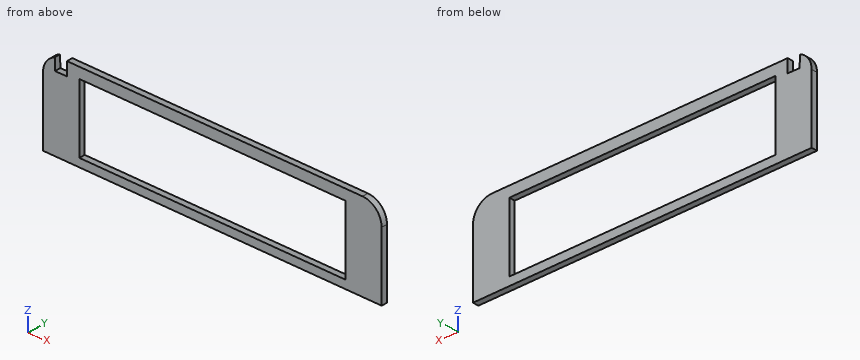
```python
from build123d import *

# Parameters (mm, degrees)
F0_W     = 70.612
F0_H     = 18.034
F1_DEPTH = 1.5748


with BuildPart() as f1:
    # F0 (on Front) → F1 (new body)
    with BuildSketch(Plane.XZ):
        with BuildLine():
            Line((43.006146, 12.59901), (-35.475917, 12.59901))
            Line((-35.475917, 12.59901), (-35.423273, 9.108076))
            Line((-35.423273, 9.108076), (-38.651996, 9.059386))
            Line((-38.651996, 9.059386), (-38.69928, 12.194926))
            ThreePointArc((-38.69928, 12.194926), (-40.974954, 10.332579), (-41.829854, 7.51901))
            Line((-41.829854, 7.51901), (-41.829854, -10.40099))
            Line((-41.829854, -10.40099), (48.086146, -10.40099))
            Line((48.086146, -10.40099), (48.086146, 7.51901))
            ThreePointArc((48.086146, 7.51901), (46.598248, 11.111112), (43.006146, 12.59901))
        make_face()
        with Locations((3.128146, 0.78801)):
            Rectangle(F0_W, F0_H, mode=Mode.SUBTRACT)
    extrude(amount=F1_DEPTH)


solid = f1.part
```
The model under review builds one solid part; all positions refer to its coordinate system, in mm. Round coordinates to 2 decimals unless told otherwise and drop trailing zeros. Loops run counter-clockwise (first coordinate to the right, second up) from the corner with the lowest first, then second, coordinate; pieces in that order, holes last. Notation, with made-up numbers: M 21,1 L 65,1 A36 ccw 65,37 Z; hole C 6,7 d4. An arc over 180 degrees is marked long. Put each result on its own line as item: value.
Q1. Consider section C-C, the plane y = -1.1. Give the boundary of the cut face in (x, z) (3 decimals), then the cut area to 3 significant figures.
Result set:
outline: M -41.83,-10.401 L 48.086,-10.401 L 48.086,7.519 A5.08 ccw 43.006,12.599 L -35.476,12.599 L -35.423,9.108 L -38.652,9.059 L -38.699,12.195 A5.057 ccw -41.83,7.519 Z; hole M -32.178,-8.229 L 38.434,-8.229 L 38.434,9.805 L -32.178,9.805 Z
area: 772 mm²
Q2. To check wall thickness, follow L1, parallel to X at y = -0.05, z = -7.5; L2, parallel to Z at x = -21, y = -1.05; L3, parallel to X at y = -0.25, z = 11.75. State the ranges of each line that lie inside material, in increasing order.
Result set:
L1: x = -41.83 to -32.18, 38.43 to 48.09
L2: z = -10.4 to -8.23, 9.81 to 12.6
L3: x = -39.54 to -38.69, -35.46 to 45.82
Q3. Consider section A-A, the plane x = 0. Give the boundary of the cut face in (y, z) (3 decimals), then the cut area to 3 significant figures.
Result set:
outline: M -1.575,-10.401 L 0,-10.401 L 0,-8.229 L -1.575,-8.229 Z; M -1.575,9.805 L 0,9.805 L 0,12.599 L -1.575,12.599 Z
area: 7.82 mm²
Q4. Consider section B-B, the plane z = 1.5. Give the boundary of the cut face in (x, y).
Result set:
outline: M -41.83,-1.57 L -32.18,-1.57 L -32.18,0 L -41.83,0 Z; M 38.43,-1.57 L 48.09,-1.57 L 48.09,0 L 38.43,0 Z
